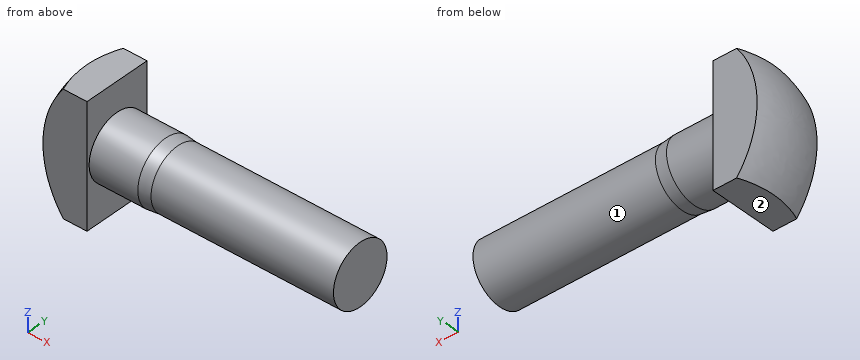
Autodesk Inventor part; units mm, degrees
ref_plane "IDS_WORKPLANE{1}" through (0, 0, 0) normal (0, 1, 0) x (-1, 0, 0)
ref_plane "Work Plane3" through (15.875, 0, 0) normal (0, 0, -1) x (1, 0, 0)
ref_plane "YZ Plane" through (0, 0, 0) normal (1, 0, 0) x (0, 1, 0)
sketch "Boceto1" plane through (0, 0, 0) normal (0, 0, 1) x (1, 0, 0)
  line L0 (0, 3.302) -> (5.08, 3.302)
  line L1 (5.08, 3.302) -> (6.35, 3.175)
  line L2 (6.35, 3.175) -> (25.4, 3.175)
  line L3 (25.4, 3.175) -> (25.4, 2.4879)
  line L4 (25.4, 2.4879) -> (25.4, 0)
  line L5 (0, 3.9624) -> (0, -0.6604)
  line L6 (0, 3.302) -> (0, 0)
  line L7 (-0.4343, 0) -> (7.5114, 0)
  line L8 (-5.6012, 0) -> (30.5669, 0)
  line L9 (0, 0) -> (25.4, 0)
  dimension "d0" = 0
  dimension "d1" = 19.05
  dimension "d2" = 1.27
  dimension "d3" = 4.9759
  dimension "d4" = 6.35
  dimension "d5" = 6.604
  dimension "d6" = 25.4
revolve "Cuerpo" add sketch "Boceto1" angle 360 about axis through (-0.4343, 0, 0) along (1, 0, 0)
sketch "Boceto2" plane through (0, 0, 0) normal (-1, 0, 0) x (0, 0, 1)
  line L0 (-6.35, 3.556) -> (6.35, 3.556)
  line L1 (6.35, 3.556) -> (6.35, -3.556)
  line L2 (6.35, -3.556) -> (-6.35, -3.556)
  line L3 (-6.35, -3.556) -> (-6.35, 3.556)
  line L4 (-8.89, 0) -> (8.89, 0)
  line L5 (0, 4.9784) -> (0, -4.9784)
  dimension "d7" = 3.556
  dimension "d8" = 7.112
  dimension "d9" = 6.35
  dimension "d10" = 12.7
extrude "Cabeza" add sketch "Boceto2" along normal blind 5.1816
ref_plane "IDS_WORKPLANE{1}" through (0, 0, 0) normal (0, 1, 0) x (-1, 0, 0)
sketch "Boceto3" plane through (0, 0, 0) normal (0, 1, 0) x (-1, 0, 0)
  arc A0 (5.1816, 0) -> (-0.1952, 9.525) centre (-5.9436, 0) ccw
  line L0 (0, -9.6663) -> (0, 13.5477)
  line L1 (8.9083, 0) -> (-8.4189, 0)
  line L2 (5.1816, 6.35) -> (5.1816, 9.525)
  line L3 (5.1816, 9.525) -> (-0.1952, 9.525)
  line L4 (5.1816, 6.35) -> (5.1816, -6.35)
  dimension "d15" = 11.1252
  dimension "d19" = 19.05
revolve "Empalme1" cut sketch "Boceto3" angle 360 about axis through (-10, 0, 0) along (1, 0, 0) contours A0 L0 L3 L2 L4 | A0 L3 L0
thread "Rosca"
ref_plane "Work Plane3" through (15.875, 0, 0) normal (0, 0, -1) x (1, 0, 0)
equation "\"d7\" = 0.5 * KBR"
equation "\"d8\" = KBR"
equation "\"d9\" = 0.5 * KOL"
equation "\"d10\" = KOL"
equation "\"d11\" = KOH"
equation "\"d15\" = KR"
equation "\"d19\" = 1.5 * KOL"
equation "\"d1\" = GEL"
equation "\"d2\" = GAL"
equation "\"d3\" = SPD"
equation "\"d4\" = GD"
equation "\"d5\" = BDM"
equation "\"d6\" = NLG"
equation "\"GD\" = NND"
equation "\"NLG\" = 25.4"
equation "\"GAL\" = 1.27"
equation "\"GEL\" = 19.05"
equation "\"BDM\" = 6.604"
equation "\"KOL\" = 12.7"
equation "\"KBR\" = 7.112"
equation "\"KOH\" = 5.1816"
equation "\"KR\" = 11.1252"
equation "\"SPD\" = GD1"
equation "\"RR\" = -0.5 * BDM + 0.5 * KBR"
equation "\"d13\" = 0.5 * KOL"
equation "\"GUL\" = 0"
equation "\"PHH\" = 0.15 * KOH"
equation "\"THREADDIA\" = 6.35"
equation "\"TOA\" = 30deg"
equation "\"NND\" = 6.35"
equation "\"GD1\" = 4.97586"
properties part number "ANSI/ASME B18.5 - 1/4 - 20 - 1" material "Acero, suave"
Check sheet for the modelled part. Datum: model origin and axes. Units: mm. Face numbers are marked on the shaded views. A direction names the side the tool comes from. Give positions to 0.01 mm unless a question says otherwise; leave off trailing zeros. Loops run counter-clockwise (first coordinate to the right, second up) from the corner with the lowest first, then second, coordinate; pieces in that order, holes last. Notation, with made-up numbers: M 1.25,83 L 37.25,83 A28 cw 37.25,111 Z; hole C 64.5,69.5 d3. An arc over 180 degrees is marked long. Use a Markdown table: item, result. Add a question column.
Q1. Tool access check on the marked faces 1 and 2. Record the directions out of +Z, -Z, +X, -X, +Y, -Y that give a thin tool (end or side, any length) a straight path to the whole face; none if there is none.
Q2. Sectioned sample at A-A, the plane x = 17.5. Record the cut outline in (y, z) (3 decimals), then the cut area to 3 significant figures.
Q3. Scan lines: line 1 along Z through (x, y) = (20.5, 0) (3 decimals); line 2 along Y through (x, z) = (21, 1.75); line 3 along X through (y, z) = (1.75, 2.5). Record each from-to range of solid material in increasing order. Write a range as [from, to].
Q4. Go/stop test with flat-tipped pins: pin 1 (2 mm diameter, centred on x = 19, y = -2, fed in from -Z); pin 2 (1.5 mm diameter, centred on x = 13.5, y = 0.5, fed in from -Z) (3 decimals). Record where each tip stops, or that it passes through.
Verdict:
| question | item | result |
|---|---|---|
| 1 | face 1 | +X |
| 1 | face 2 | -Z, +X, -X, +Y, -Y |
| 2 | outline | C 0,0 d6.35 |
| 2 | area | 31.7 mm^2 |
| 3 | line 1 | [-3.175, 3.175] |
| 3 | line 2 | [-2.65, 2.65] |
| 3 | line 3 | [-4.75, 25.4] |
| 4 | pin 1 | z = -3.01 |
| 4 | pin 2 | z = -3.175 |
